Work out the finished part from the listing and answer in its coordinate system (mm). Face numbers are marked on the shaded views. Coordinates: 2 decimals unless noted, no trailing zeros. Loops run counter-clockwise (first coordinate to the right, second up) from the corner with the lowest first, then second, coordinate; pieces in that order, holes last. Notation, with made-up numbers: (-30, -8) -> (-21, -8) arc R23 ccw to (-21, 5) -> close; hole circle Ø10 at (-12.75, 54.25). An arc over 180 degrees is marked (long way). Answer as CSV lines item,"result".
```python
from build123d import *

# Parameters (mm, degrees)
SKETCH1_R           = 4.7625
BOSS_EXTRUDE1_DEPTH = 9.525
BOSS_EXTRUDE4_START = 25.4
SKETCH4_R           = 4.7625
BOSS_EXTRUDE4_DEPTH = 25.4


with BuildPart() as part:
    # Sketch1 → Boss-Extrude1 (new body)
    with BuildSketch(Plane.XY):
        with BuildLine():
            ThreePointArc((0, 9.525), (-9.525, 0), (0, -9.525))
            Line((0, -9.525), (1.770377541, -9.359027106))
            Line((1.770377541, -9.359027106), (50.8, -4.7625))
            ThreePointArc((50.8, -4.7625), (55.5625, 0), (50.8, 4.7625))
            Line((50.8, 4.7625), (1.770377541, 9.359027106))
            Line((1.770377541, 9.359027106), (0, 9.525))
        make_face()
        with Locations(Location((0, 0, 0), (0, 0, 180))):
            Circle(SKETCH1_R, mode=Mode.SUBTRACT)
    extrude(amount=BOSS_EXTRUDE1_DEPTH)

    # Sketch4 → Boss-Extrude4 (add)
    with BuildSketch(Plane(origin=(0, 0, 0), x_dir=(-1, 0, 0), z_dir=(0, 0, -1)).offset(BOSS_EXTRUDE4_START)):
        with Locations((-50.8, 0)):
            Circle(SKETCH4_R)
    extrude(amount=-BOSS_EXTRUDE4_DEPTH)


solid = part.part
```
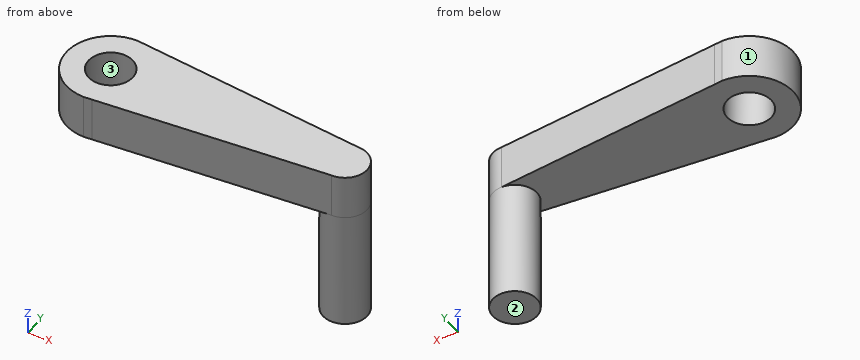
(1) A cutting plane is placed at B-B, the plane x = -1. Write down the section's boundary in (y, z) (3 decimals).
Computed values:
outline,"(-9.472, 0) -> (-4.656, 0) -> (-4.656, 9.525) -> (-9.472, 9.525) -> close; (4.656, 0) -> (9.472, 0) -> (9.472, 9.525) -> (4.656, 9.525) -> close"
(2) Consider line 1 along Y through (x, z) = (51, -2.5); line 2 along X through (y, z) = (-1.5, 1); line 3 along X through (y, z) = (-0.5, 6). Determine where each line is inside the solid, lowest interval first.
Computed values:
line 1,"-4.76 to 4.76"
line 2,"-9.41 to -4.52, 4.52 to 55.32"
line 3,"-9.51 to -4.74, 4.74 to 55.54"
(3) Flat-ended cylindrical pins translate along their axes: pin 1 Ø2 at (x, y) = (20.5, -2.5) entering from -Z; pin 2 Ø5 at (y, z) = (6, 0.5) entering from -X; pin 3 Ø8 at (y, z) = (-5.5, -21.5) entering from -X. Find the tip coordinate at first contact, or state that the pin passes through.
Computed values:
pin 1,"z = 0"
pin 2,"x = -8.86"
pin 3,"x = 46.28"
(4) A cutting plane is placed at A-A, the plane y = 0. Write down the section's boundary in (x, z) (1 decimal), and give its area (3 significant figures).
Computed values:
outline,"(-9.5, 0) -> (-4.8, 0) -> (-4.8, 9.5) -> (-9.5, 9.5) -> close; (4.8, 0) -> (46, 0) -> (46, -25.4) -> (55.6, -25.4) -> (55.6, 9.5) -> (4.8, 9.5) -> close"
area,"771 mm2"
(5) A cutting plane is placed at D-D, the plane y = -3. Write down the section's boundary in (x, z) (3 decimals), and give its area (3 significant figures).
Computed values:
outline,"(-9.04, 0) -> (-3.699, 0) -> (-3.699, 9.525) -> (-9.04, 9.525) -> close; (3.699, 0) -> (47.101, 0) -> (47.101, -25.4) -> (54.499, -25.4) -> (54.499, 9.525) -> (3.699, 9.525) -> close"
area,"723 mm2"
(6) A cutting plane is placed at C-C, the plane z = -20. Write down the section's boundary in (x, y) (1 decimal), and give its area (3 significant figures).
Computed values:
outline,"circle Ø9.5 at (50.8, 0)"
area,"71.3 mm2"
(7) For a pull along X with two mould halves and no side action, classify the marked faces 1, 2 and 3 as pulls with the +X half, pulls with the -X half, needs draft (parallel to the pull), parting line crosses it, or undercut.
Computed values:
face 1,"pulls with the -X half"
face 2,"needs draft"
face 3,"undercut"
